Part model, mm, in its own coordinate system. Face numbers are marked on the shaded views. A direction names the side the tool comes from. Coordinates: 2 decimals unless noted, no trailing zeros. Write each loop counter-clockwise with the first axis right and the second up, starting at its lowest first coordinate (ties: lowest second). Pieces come first, ordered by that corner, then holes. Notation, with made-up numbers: (75.5, 68) -> (101.5, 68) arc R19 ccw to (101.5, 105) -> close; hole circle Ø4 at (52.25, 43). An arc over 180 degrees is marked (long way). One line per question, with ' | ' between items. Start each with the question number.
Item 1: Probe probe 1 along Z at (x, y) = (15, -25.5); probe 2 along X at (y, z) = (-9, 18.5); probe 3 along Y at (x, z) = (4.5, 22.25). List the from-to ranges inside material, lowest first. Write a range as [from, to].
Item 2: Saw through at D-D (y = -8). List the corners of the cut face in (x, z), and give its area (3 significant figures).
Item 3: Saw through at A-A (z = 14.5). List the corners of the cut face in (x, y), and give its area (3 significant figures).
Item 4: Saw through at C-C (x = -2). List the corners of the cut face in (y, z), and give its area (3 significant figures).
Item 5: 3-axis set-ups, long thin cutter, end or side, ignore diameter. For the marked faces 4, 5, 6 and 7: which of +Z, -Z, +X, -X, +Y, -Y reach the whole face in a straight line?
Item 6: Saw through at B-B (y = -27.5). List the corners of the cut face in (x, z).
Item 7: Pin check, flat tips, straight feed: pin 1 (3 mm diameter, centred on x = -18, y = -20, fed in from +Z); pin 2 (1.2 mm diameter, centred on y = -1.5, z = 21, fed in from -X); pin 3 (17.5 mm diameter, centred on x = -1.56, y = -9.18, fed in from +Z); pin 4 (1.2 mm diameter, centred on x = 1, y = -1, fed in from +Z). Stop position of each tip, or through.
Item 8: Two-plate mould, pull along X, no slides. Class the marked faces 1, 2 and 3: pulls with the +X half, pulls with the -X half, needs draft (parallel to the pull), parting line crosses it, or undercut.
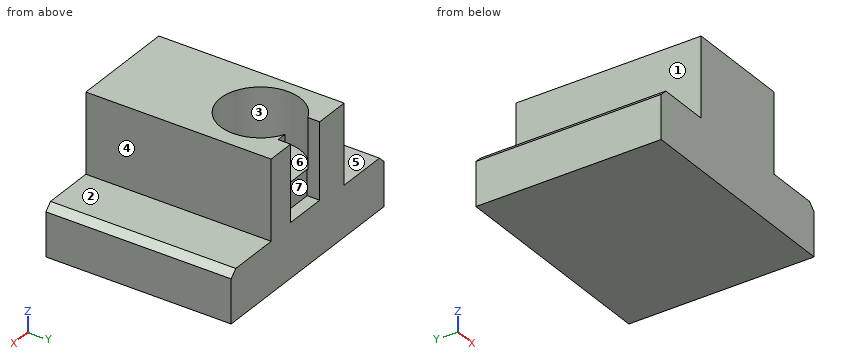
from build123d import *

# Parameters (mm, degrees)
F1_DEPTH = 35.0012
F2_R     = 7.5311
F3_DEPTH = 24.638
F4_DEPTH = 15.0622
F5_W     = 7.9995468259
F5_H     = 14.370085096
F6_DEPTH = 2.3622
F7_SIZE  = 1.27


# Not quite as in the source:
# - a feature names something its author has since deleted; it is built from what else it names


with BuildPart() as f1:
    # F0 (on Front) → F1 (new body)
    with BuildSketch(Plane.XZ):
        Polygon((-22.2087535855, 0), (-22.0162163296, 0), (19.8619475364, 0), (19.8619475364, 9.5335517829), (8.8637475364, 9.5335517829), (8.8637475364, 24.5957517829), (-11.2105535855, 24.5957517829), (-11.2105535855, 9.5335517829), (-22.2087535855, 9.5335517829), align=None)
    extrude(amount=F1_DEPTH)

    # F2 (on Top) → F3 (cut)
    with BuildSketch(Plane.XY):
        with Locations((-1.5582955675, -9.1819977388)):
            Circle(F2_R)
    extrude(amount=F3_DEPTH, mode=Mode.SUBTRACT)

    # F2 (on Top) → F4 (join)
    with BuildSketch(Plane.XY):
        with Locations((-1.5582955675, -9.1819977388)):
            Circle(F2_R)
    extrude(amount=F4_DEPTH)

    # F5 (on face) → F6 (cut, symmetric)
    with BuildSketch(Plane.XZ):
        with Locations((-0.500776805, 17.4107092349)):
            Rectangle(F5_W, F5_H)
    extrude(amount=F6_DEPTH, both=True, mode=Mode.SUBTRACT)

    # F7
    f7_edges = [f1.edges().sort_by_distance(p)[0] for p in [
        (19.861948, -17.5006, 9.533552),
        (-22.208754, -17.5006, 9.533552),
    ]]
    chamfer(f7_edges, length=F7_SIZE)


solid = f1.part
From the geometry:
1) probe 1: [0, 9.53] | probe 2: [-11.21, -9.09], [5.97, 8.86] | probe 3: [-35, -13.66], [-4.71, 0]
2) outline: (-22.21, 0) -> (19.86, 0) -> (19.86, 8.26) -> (18.59, 9.53) -> (8.86, 9.53) -> (8.86, 24.6) -> (5.88, 24.6) -> (5.88, 15.06) -> (-9, 15.06) -> (-9, 24.6) -> (-11.21, 24.6) -> (-11.21, 9.53) -> (-20.94, 9.53) -> (-22.21, 8.26) -> close | area: 560 mm2
3) outline: (-11.21, -35) -> (8.86, -35) -> (8.86, 0) -> (3.5, 0) -> (3.5, -2.36) -> (-4.5, -2.36) -> (-4.5, 0) -> (-11.21, 0) -> close | area: 684 mm2
4) outline: (-35, 0) -> (0, 0) -> (0, 10.23) -> (-2.36, 10.23) -> (-2.36, 15.06) -> (-16.7, 15.06) -> (-16.7, 24.6) -> (-35, 24.6) -> close | area: 690 mm2
5) face 4: +Z, +X, +Y, -Y | face 5: +Z, -X, +Y, -Y | face 6: +Z | face 7: +Z, +Y
6) outline: (-22.21, 0) -> (19.86, 0) -> (19.86, 8.26) -> (18.59, 9.53) -> (8.86, 9.53) -> (8.86, 24.6) -> (-11.21, 24.6) -> (-11.21, 9.53) -> (-20.94, 9.53) -> (-22.21, 8.26) -> close
7) pin 1: z = 9.53 | pin 2: x = -11.21 | pin 3: z = 24.6 | pin 4: z = 10.23
8) face 1: pulls with the -X half | face 2: needs draft | face 3: undercut
